The listing builds one solid part. Answer for the finished solid, in the listing's coordinates (mm). Face numbers are marked on the shaded views. A direction names the side the tool comes from. Coordinates: 2 decimals unless noted, no trailing zeros. Write each loop counter-clockwise with the first axis right and the second up, starting at its lowest first coordinate (ties: lowest second). Pieces come first, ordered by that corner, then holes. Notation, with made-up numbers: M -14.5,78.25 L 18.5,78.25 A17 ccw 18.5,86.25 Z; hole C 0,-27 d3. An arc over 180 degrees is marked long. Answer as CSV lines item,"result". Start each with the question number.
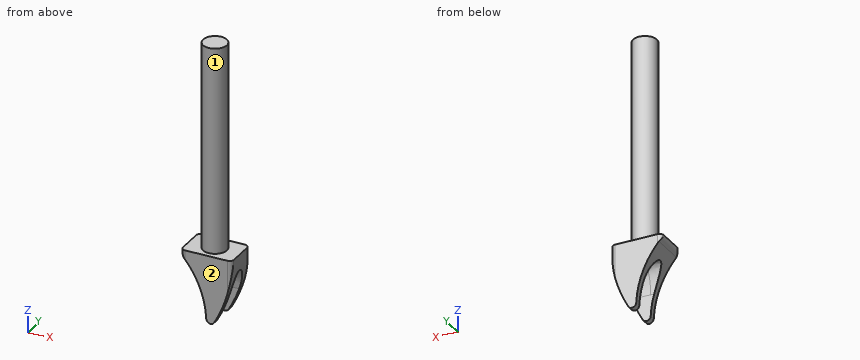
```python
from build123d import *

# Parameters (mm, degrees)
F0_R     = 14
F1_DEPTH = 244
F2_W     = 60
F2_H     = 40
F3_DEPTH = 80
F4_R     = 5
F6_DEPTH = 40
F8_DEPTH = 35


with BuildPart() as f1:
    # F0 (on Top) → F1 (new body)
    with BuildSketch(Plane.XY):
        Circle(F0_R)
    extrude(amount=F1_DEPTH)

    # F2 (on Top) → F3 (join)
    with BuildSketch(Plane.XY):
        Rectangle(F2_W, F2_H)
    extrude(amount=-F3_DEPTH)

    # F4
    f4_edges = [f1.edges().sort_by_distance(p)[0] for p in [
        (30, -20, -40),
        (-30, -20, -40),
        (30, 20, -40),
        (-30, 20, -40),
    ]]
    fillet(f4_edges, radius=F4_R)

    # F5 (on Front) → F6 (cut, symmetric)
    with BuildSketch(Plane.XZ):
        with BuildLine():
            Line((-30, 0), (-30, -90))
            Line((-30, -90), (30, -90))
            Line((30, -90), (30, 0))
            ThreePointArc((30, 0), (24.7453124754, -40.0987499935), (9.3360995851, -77.489626556))
            ThreePointArc((9.3360995851, -77.489626556), (3.8189128101, -79.8585011114), (0.0048970649, -75.2212389381))
            ThreePointArc((0.0048970649, -75.2212389381), (-7.6784593534, -39.7286436891), (-26.6918835796, -8.7892192835))
            ThreePointArc((-26.6918835796, -8.7892192835), (-29.1455882011, -4.6955832935), (-30, 0))
        make_face()
    extrude(amount=F6_DEPTH, both=True, mode=Mode.SUBTRACT)

    # F7 (on Right) → F8 (cut, symmetric)
    with BuildSketch(Plane.YZ):
        with BuildLine():
            Line((13, -80), (13, -50))
            add(Edge.make_bspline(
                [(13, -50), (13, -20), (0, -20), (-13, -20), (-13, -50)],
                knots=[1.5707963268, 1.5707963268, 1.5707963268, 3.1415926536, 3.1415926536, 4.7123889804, 4.7123889804, 4.7123889804], degree=2, weights=[1, 0.7071067812, 1, 0.7071067812, 1]))
            Line((-13, -50), (-13, -80))
            Line((-13, -80), (13, -80))
        make_face()
    extrude(amount=F8_DEPTH, both=True, mode=Mode.SUBTRACT)


solid = f1.part
```
1) Which of the six approach directions +Z, -Z, +X, -X, +Y, -Y give full straight-line access (tool end or side, diameter ignored) to the marked faces 1 and 2?
2) Find the intervals of material crossed by line 1 (Y direction, x = 5.5, z = -57.5); line 2 (Y direction, x = 12.5, z = -34.5); line 3 (X direction, y = 13, z = 197), in increasing order. Write a range as from..to.
3) Each of these flat-tipped pins is pushed along its axis until it touches: P1, Ø1.5, axis at y = 5.5, z = 132.5, coming from the -X side; P2, Ø6, axis at y = 10, z = 12.5, coming from the +X side; P3, Ø3, axis at y = -12, z = 49, coming from the -X side. Where does it stop, or does it pass through?
4) The part is cut by section A-A (z = 141). Determine the outline of the cut face in (x, y), then the cut area to 3 significant figures.
Completed:
1,face 1,"+Z"
1,face 2,"+Z, -Z, +X, -X, -Y"
2,line 1,"-20..-13, 13..20"
2,line 2,"-20..-11.13, 11.13..20"
2,line 3,"-5.2..5.2"
3,P1,"x = -13.17"
3,P2,"x = 12.12"
3,P3,"x = -9.26"
4,outline,"C 0,0 d28"
4,area,"616 mm²"
